```python
from build123d import *

# Parameters (mm, degrees)
F0_R     = 1.5
F0_W     = 36
F0_H     = 85
F1_DEPTH = 4
F2_SIZE  = 10
F3_DEPTH = 7


with BuildPart() as f1:
    # F0 (on Front) → F1 (new body)
    with BuildSketch(Plane.XZ):
        Polygon((42.5, 32.5), (42.5, 42.5), (37.5, 37.5), align=None)
        Polygon((37.5, 37.5), (42.5, 42.5), (32.5, 42.5), align=None)
        Polygon((42.5, -32.5), (42.5, 32.5), (37.5, 37.5), (32.5, 42.5), (18, 42.5), (18, -42.5), (32.5, -42.5), (37.5, -37.5), align=None)
        with Locations((26.8933982822, -33.9644660941)):
            Circle(F0_R, mode=Mode.SUBTRACT)
        with BuildLine():
            ThreePointArc((35.4644660941, -33.9644660941), (35.3502853928, -34.5384912426), (35.0251262658, -35.0251262658))
            ThreePointArc((35.0251262658, -35.0251262658), (32.9038059223, -35.0251262658), (32.9038059223, -32.9038059223))
            ThreePointArc((32.9038059223, -32.9038059223), (34.5384912426, -32.5786467953), (35.4644660941, -33.9644660941))
        make_face(mode=Mode.SUBTRACT)
        with Locations((33.9644660941, -26.8933982822)):
            Circle(F0_R, mode=Mode.SUBTRACT)
        Polygon((20.7055291533, -3.823871389), (35.7055291533, -3.823871389), (35.7055291533, -18.823871389), align=None, mode=Mode.SUBTRACT)
        Polygon((35.7055291533, 3.823871389), (20.7055291533, 3.823871389), (35.7055291533, 18.823871389), align=None, mode=Mode.SUBTRACT)
        with BuildLine():
            ThreePointArc((35.4644660941, 26.8933982822), (33.3904409455, 25.5075789834), (32.9038059223, 27.954058454))
            ThreePointArc((32.9038059223, 27.954058454), (34.5384912426, 28.279217581), (35.4644660941, 26.8933982822))
        make_face(mode=Mode.SUBTRACT)
        with BuildLine():
            ThreePointArc((28.3933982822, 33.9644660941), (28.279217581, 33.3904409455), (27.954058454, 32.9038059223))
            ThreePointArc((27.954058454, 32.9038059223), (25.5075789834, 34.5384912426), (28.3933982822, 33.9644660941))
        make_face(mode=Mode.SUBTRACT)
        with BuildLine():
            ThreePointArc((32.9038059223, 32.9038059223), (32.9038059223, 35.0251262658), (35.0251262658, 35.0251262658))
            ThreePointArc((35.0251262658, 35.0251262658), (35.3502853928, 34.5384912426), (35.4644660941, 33.9644660941))
            ThreePointArc((35.4644660941, 33.9644660941), (34.5384912426, 32.5786467953), (32.9038059223, 32.9038059223))
        make_face(mode=Mode.SUBTRACT)
        Polygon((42.5, -42.5), (42.5, -32.5), (37.5, -37.5), align=None)
        Rectangle(F0_W, F0_H)
        Polygon((32.5, -42.5), (42.5, -42.5), (37.5, -37.5), align=None)
        Polygon((-18, -42.5), (-18, 42.5), (-32.5, 42.5), (-37.5, 37.5), (-42.5, 32.5), (-42.5, -32.5), (-37.5, -37.5), (-32.5, -42.5), align=None)
        with BuildLine():
            ThreePointArc((-32.4644660941, -33.9644660941), (-33.3904409455, -35.3502853928), (-35.0251262658, -35.0251262658))
            ThreePointArc((-35.0251262658, -35.0251262658), (-35.0251262658, -32.9038059223), (-32.9038059223, -32.9038059223))
            ThreePointArc((-32.9038059223, -32.9038059223), (-32.5786467953, -33.3904409455), (-32.4644660941, -33.9644660941))
        make_face(mode=Mode.SUBTRACT)
        with Locations((-26.8933982822, -33.9644660941)):
            Circle(F0_R, mode=Mode.SUBTRACT)
        with Locations((-33.9644660941, -26.8933982822)):
            Circle(F0_R, mode=Mode.SUBTRACT)
        Polygon((-20.7055291533, -3.823871389), (-35.7055291533, -18.823871389), (-35.7055291533, -3.823871389), align=None, mode=Mode.SUBTRACT)
        Polygon((-35.7055291533, 3.823871389), (-35.7055291533, 18.823871389), (-20.7055291533, 3.823871389), align=None, mode=Mode.SUBTRACT)
        with BuildLine():
            ThreePointArc((-32.7795228992, 27.2231633162), (-35.6780717969, 26.6808894181), (-33.1716042066, 28.2343587329))
            ThreePointArc((-33.1716042066, 28.2343587329), (-32.8809740014, 27.7654372144), (-32.7795228992, 27.2231633162))
        make_face(mode=Mode.SUBTRACT)
        with BuildLine():
            ThreePointArc((-32.9038059223, 32.9038059223), (-35.0251262658, 32.9038059223), (-35.0251262658, 35.0251262658))
            ThreePointArc((-35.0251262658, 35.0251262658), (-33.3904409455, 35.3502853928), (-32.4644660941, 33.9644660941))
            ThreePointArc((-32.4644660941, 33.9644660941), (-32.5786467953, 33.3904409455), (-32.9038059223, 32.9038059223))
        make_face(mode=Mode.SUBTRACT)
        with BuildLine():
            ThreePointArc((-25.3933982822, 33.9644660941), (-26.3511243841, 32.5659171963), (-28.0013169747, 32.9532706774))
            ThreePointArc((-28.0013169747, 32.9532706774), (-27.4356721803, 35.3630149918), (-25.3933982822, 33.9644660941))
        make_face(mode=Mode.SUBTRACT)
        Polygon((-37.5, 37.5), (-32.5, 42.5), (-42.5, 42.5), align=None)
        Polygon((-42.5, 32.5), (-37.5, 37.5), (-42.5, 42.5), align=None)
        Polygon((-42.5, -42.5), (-32.5, -42.5), (-37.5, -37.5), align=None)
        Polygon((-42.5, -42.5), (-37.5, -37.5), (-42.5, -32.5), align=None)
    extrude(amount=F1_DEPTH)

    # F2
    f2_edges = [f1.edges().sort_by_distance(p)[0] for p in [
        (42.5, -2, 42.5),
        (-42.5, -2, 42.5),
        (-42.5, -2, -42.5),
        (42.5, -2, -42.5),
    ]]
    chamfer(f2_edges, length=F2_SIZE)

    # F0 (on Front) → F3 (join)
    with BuildSketch(Plane.XZ):
        Polygon((-18, -42.5), (-18, 42.5), (-32.5, 42.5), (-37.5, 37.5), (-42.5, 32.5), (-42.5, -32.5), (-37.5, -37.5), (-32.5, -42.5), align=None)
        with BuildLine():
            ThreePointArc((-32.4644660941, -33.9644660941), (-33.3904409455, -35.3502853928), (-35.0251262658, -35.0251262658))
            ThreePointArc((-35.0251262658, -35.0251262658), (-35.0251262658, -32.9038059223), (-32.9038059223, -32.9038059223))
            ThreePointArc((-32.9038059223, -32.9038059223), (-32.5786467953, -33.3904409455), (-32.4644660941, -33.9644660941))
        make_face(mode=Mode.SUBTRACT)
        with Locations((-26.8933982822, -33.9644660941)):
            Circle(F0_R, mode=Mode.SUBTRACT)
        with Locations((-33.9644660941, -26.8933982822)):
            Circle(F0_R, mode=Mode.SUBTRACT)
        Polygon((-20.7055291533, -3.823871389), (-35.7055291533, -18.823871389), (-35.7055291533, -3.823871389), align=None, mode=Mode.SUBTRACT)
        Polygon((-35.7055291533, 3.823871389), (-35.7055291533, 18.823871389), (-20.7055291533, 3.823871389), align=None, mode=Mode.SUBTRACT)
        with BuildLine():
            ThreePointArc((-32.7795228992, 27.2231633162), (-35.6780717969, 26.6808894181), (-33.1716042066, 28.2343587329))
            ThreePointArc((-33.1716042066, 28.2343587329), (-32.8809740014, 27.7654372144), (-32.7795228992, 27.2231633162))
        make_face(mode=Mode.SUBTRACT)
        with BuildLine():
            ThreePointArc((-32.9038059223, 32.9038059223), (-35.0251262658, 32.9038059223), (-35.0251262658, 35.0251262658))
            ThreePointArc((-35.0251262658, 35.0251262658), (-33.3904409455, 35.3502853928), (-32.4644660941, 33.9644660941))
            ThreePointArc((-32.4644660941, 33.9644660941), (-32.5786467953, 33.3904409455), (-32.9038059223, 32.9038059223))
        make_face(mode=Mode.SUBTRACT)
        with BuildLine():
            ThreePointArc((-25.3933982822, 33.9644660941), (-26.3511243841, 32.5659171963), (-28.0013169747, 32.9532706774))
            ThreePointArc((-28.0013169747, 32.9532706774), (-27.4356721803, 35.3630149918), (-25.3933982822, 33.9644660941))
        make_face(mode=Mode.SUBTRACT)
        Polygon((42.5, -32.5), (42.5, 32.5), (37.5, 37.5), (32.5, 42.5), (18, 42.5), (18, -42.5), (32.5, -42.5), (37.5, -37.5), align=None)
        with Locations((26.8933982822, -33.9644660941)):
            Circle(F0_R, mode=Mode.SUBTRACT)
        with BuildLine():
            ThreePointArc((35.4644660941, -33.9644660941), (35.3502853928, -34.5384912426), (35.0251262658, -35.0251262658))
            ThreePointArc((35.0251262658, -35.0251262658), (32.9038059223, -35.0251262658), (32.9038059223, -32.9038059223))
            ThreePointArc((32.9038059223, -32.9038059223), (34.5384912426, -32.5786467953), (35.4644660941, -33.9644660941))
        make_face(mode=Mode.SUBTRACT)
        with Locations((33.9644660941, -26.8933982822)):
            Circle(F0_R, mode=Mode.SUBTRACT)
        Polygon((20.7055291533, -3.823871389), (35.7055291533, -3.823871389), (35.7055291533, -18.823871389), align=None, mode=Mode.SUBTRACT)
        Polygon((35.7055291533, 3.823871389), (20.7055291533, 3.823871389), (35.7055291533, 18.823871389), align=None, mode=Mode.SUBTRACT)
        with BuildLine():
            ThreePointArc((35.4644660941, 26.8933982822), (33.3904409455, 25.5075789834), (32.9038059223, 27.954058454))
            ThreePointArc((32.9038059223, 27.954058454), (34.5384912426, 28.279217581), (35.4644660941, 26.8933982822))
        make_face(mode=Mode.SUBTRACT)
        with BuildLine():
            ThreePointArc((28.3933982822, 33.9644660941), (28.279217581, 33.3904409455), (27.954058454, 32.9038059223))
            ThreePointArc((27.954058454, 32.9038059223), (25.5075789834, 34.5384912426), (28.3933982822, 33.9644660941))
        make_face(mode=Mode.SUBTRACT)
        with BuildLine():
            ThreePointArc((32.9038059223, 32.9038059223), (32.9038059223, 35.0251262658), (35.0251262658, 35.0251262658))
            ThreePointArc((35.0251262658, 35.0251262658), (35.3502853928, 34.5384912426), (35.4644660941, 33.9644660941))
            ThreePointArc((35.4644660941, 33.9644660941), (34.5384912426, 32.5786467953), (32.9038059223, 32.9038059223))
        make_face(mode=Mode.SUBTRACT)
    extrude(amount=F3_DEPTH)


solid = f1.part
```
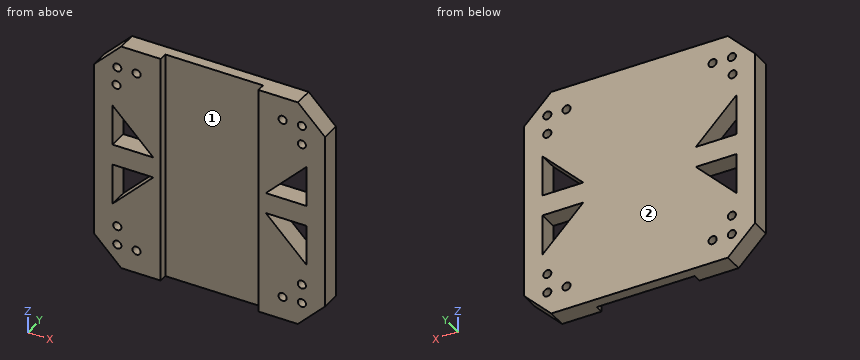
Check sheet for the modelled part. Datum: model origin and axes. Units: mm. Face numbers are marked on the shaded views. Round coordinates to 2 decimals unless told otherwise and drop trailing zeros. Order: outer loops, then holes, each group sorted by start corner. A loop starts at its lowest first (then second) coordinate and runs counter-clockwise, first axis right, second up.
1) Go/stop test with flat-tipped pins: pin 1 Ø2.5 at (x, z) = (-26.89, -33.96) entering from -Y; pin 2 Ø5 at (x, z) = (23.5, -5.5) entering from -Y; pin 3 Ø10 at (x, z) = (-2.5, -29.5) entering from -Y. Record where each tip stops, or that it passes through.
2) Section check C-C (x = 34). Record the boundary of the cut face in (y, z), and give its area (3 significant figures).
3) Section check D-D (z = -15). Record the boundary of the cut face in (x, y).
4) Section check A-A (x = 22.5). Record the boundary of the cut face in (y, z), and give its area (3 significant figures).
5) Section check B-B (z = 16.5). Record the boundary of the cut face in (x, y).
6) Scan lines: line 1 (Z direction, x = 28, y = -2.25); line 2 (Z direction, x = 27, y = -4); line 3 (X direction, y = -6, z = -21.5). Record each from-to range of solid material in increasing order.
7) Mould release check, pull along X, two halves, no side actions. Record for the marked faces 1 and 2: +X half, -X half, draft (parallel to the pull), parting line (faces both ways), or undercut.
Result:
1. pin 1: passes through
1. pin 2: stops at y = -7
1. pin 3: stops at y = -4
2. outline: (-7, -41) - (0, -41) - (0, -35.46) - (-7, -35.46) - close; (-7, -32.46) - (0, -32.46) - (0, -28.39) - (-7, -28.39) - close; (-7, -25.39) - (0, -25.39) - (0, -17.12) - (-7, -17.12) - close; (-7, -3.82) - (0, -3.82) - (0, 3.82) - (-7, 3.82) - close; (-7, 17.12) - (0, 17.12) - (0, 25.39) - (-7, 25.39) - close; (-7, 28.39) - (0, 28.39) - (0, 32.46) - (-7, 32.46) - close; (-7, 35.46) - (0, 35.46) - (0, 41) - (-7, 41) - close
2. area: 304 mm2
3. outline: (-42.5, -7) - (-35.71, -7) - (-35.71, 0) - (-42.5, 0) - close; (-31.88, -7) - (-18, -7) - (-18, -4) - (18, -4) - (18, -7) - (31.88, -7) - (31.88, 0) - (-31.88, 0) - close; (35.71, -7) - (42.5, -7) - (42.5, 0) - (35.71, 0) - close
4. outline: (-7, -42.5) - (0, -42.5) - (0, -5.62) - (-7, -5.62) - close; (-7, -3.82) - (0, -3.82) - (0, 3.82) - (-7, 3.82) - close; (-7, 5.62) - (0, 5.62) - (0, 42.5) - (-7, 42.5) - close
4. area: 570 mm2
5. outline: (-42.5, -7) - (-35.71, -7) - (-35.71, 0) - (-42.5, 0) - close; (-33.38, -7) - (-18, -7) - (-18, -4) - (18, -4) - (18, -7) - (33.38, -7) - (33.38, 0) - (-33.38, 0) - close; (35.71, -7) - (42.5, -7) - (42.5, 0) - (35.71, 0) - close
6. line 1: z = -42.5 to -34.98, -32.95 to -11.12, -3.82 to 3.82, 11.12 to 32.95, 34.98 to 42.5
6. line 2: z = -42.5 to -35.46, -32.47 to -10.12, -3.82 to 3.82, 10.12 to 32.47, 35.46 to 42.5
6. line 3: x = -42.5 to -18, 18 to 42.5
7. face 1: undercut
7. face 2: draft
